Autodesk Inventor part; units mm, degrees
ref_plane "YZ Plane" through (0, 0, 0) normal (1, 0, 0) x (0, 1, 0)
ref_plane "XZ Plane" through (0, 0, 0) normal (0, 1, 0) x (-1, 0, 0)
ref_plane "XY Plane" through (0, 0, 0) normal (0, 0, 1) x (1, 0, 0)
sketch "Sketch1" plane through (0, 0, 0) normal (0, 1, 0) x (-1, 0, 0)
  line L0 (0, -23.3131) -> (0, 24.6505)
  line L1 (49.2542, 0) -> (-47.6933, 0)
  arc A0 (37.265, -6.345) -> (37.265, -10.765) centre (35.3109, -8.555) ccw
  line L2 (37.265, -14.815) -> (37.265, -10.765)
  arc A1 (37.265, 10.765) -> (37.265, 6.345) centre (35.3109, 8.555) ccw
  line L3 (37.265, 14.815) -> (37.265, 10.765)
  line L4 (37.265, -6.345) -> (37.265, 6.345)
  line L5 (37.265, -14.815) -> (29.695, -14.815)
  line L6 (37.265, 14.815) -> (29.695, 14.815)
  arc A2 (-37.265, -10.765) -> (-37.265, -6.345) centre (-35.3109, -8.555) ccw
  line L7 (-37.265, -14.815) -> (-37.265, -10.765)
  line L8 (-37.265, 14.815) -> (-37.265, 10.765)
  arc A3 (-37.265, 6.345) -> (-37.265, 10.765) centre (-35.3109, 8.555) ccw
  line L9 (-37.265, -6.345) -> (-37.265, 6.345)
  line L10 (-37.265, -14.815) -> (-29.695, -14.815)
  line L11 (-37.265, 14.815) -> (-29.695, 14.815)
  line L12 (29.695, -14.815) -> (-29.695, -14.815)
  line L13 (-29.695, 14.815) -> (29.695, 14.815)
  line L14 (29.695, -14.815) -> (29.695, 14.815)
  line L15 (-29.695, -14.815) -> (-29.695, 14.815)
  point P0 (0, 0)
  dimension "d3" = 4.42
  dimension "d6" = 2.95
  dimension "d7" = 7.57
  dimension "d8" = 3.31
  dimension "d9" = 59.39
  dimension "d10" = 29.63
extrude "Extrusion1" add sketch "Sketch1" along normal blind 3.95
sketch "Sketch2" plane through (0, 3.95, 0) normal (0, 1, 0) x (1, 0, 0)
  line L0 (37.265, 14.815) -> (-37.265, 14.815)
  line L1 (-37.265, -14.815) -> (37.265, -14.815)
  line L2 (-29.695, 14.815) -> (29.695, 14.815)
  line L3 (29.695, 14.815) -> (29.695, -14.815)
  line L4 (29.695, -14.815) -> (-29.695, -14.815)
  line L5 (-29.695, -14.815) -> (-29.695, 14.815)
  point P0 (0, 0)
  dimension "d13" = 59.39
  dimension "d14" = 29.695
extrude "Extrusion2" add sketch "Sketch2" along normal blind 3.5
sketch "Sketch3" plane through (0, 0, 0) normal (0, -1, 0) x (1, 0, 0)
  line L0 (37.265, -14.815) -> (-37.265, -14.815)
  line L1 (-37.265, 14.815) -> (37.265, 14.815)
  line L2 (-29.695, 14.815) -> (29.695, 14.815)
  line L3 (29.695, 14.815) -> (29.695, -14.815)
  line L4 (29.695, -14.815) -> (-29.695, -14.815)
  line L5 (-29.695, -14.815) -> (-29.695, 14.815)
  point P0 (0, 0)
  dimension "d17" = 59.39
  dimension "d18" = 29.695
extrude "Extrusion3" add sketch "Sketch3" along normal blind 49.69
sketch "Sketch4" plane through (37.265, 0, 14.815) normal (0, 0, 1) x (1, 0, 0)
  line L0 (-7.57, -49.69) -> (-66.96, -49.69)
  line L1 (-66.96, 7.45) -> (-7.57, 7.45)
  line L2 (-74.53, 0) -> (-74.53, 3.95)
  line L3 (-66.96, 7.45) -> (-55.11, 10.31)
  line L4 (-55.11, 10.31) -> (-19.42, 10.31)
  line L5 (-19.42, 10.31) -> (-7.57, 7.45)
  line L6 (14.6439, 12.17) -> (-93.8376, 12.17) construction
  line L7 (-75.1527, 11.11) -> (-5.1295, 11.11) construction
  point P0 (-37.265, 0)
  dimension "d21" = 11.85
  dimension "d22" = 11.85
  dimension "d31" = 1.06
  dimension "d32" = 0.8
  dimension "d44" = 60.8
sketch "Sketch5" plane through (0, 7.45, 0) normal (0, 1, 0) x (1, 0, 0)
  line L0 (29.695, -14.815) -> (29.695, 14.815)
  line L1 (29.695, 14.815) -> (-29.695, 14.815)
  circle A0 centre (17.845, 0) radius 9
  point P0 (0, 0)
  dimension "d23" = 11.85
  dimension "d24" = 18
  dimension "d29" = 14.815
extrude "Extrusion4" add sketch "Sketch5" along normal blind 4.72
sketch "Sketch6" plane through (0, 7.45, 0) normal (0, 1, 0) x (1, 0, 0)
  line L0 (-29.695, 14.815) -> (-29.695, -14.815)
  line L1 (-22.695, 12.5) -> (3.505, 12.5)
  line L2 (3.505, 12.5) -> (3.505, -12.5)
  line L3 (3.505, -12.5) -> (-22.695, -12.5)
  line L4 (-22.695, -12.5) -> (-22.695, 12.5)
  line L5 (-37.265, 6.345) -> (-37.265, -6.345)
  point P0 (0, 0)
  dimension "d35" = 25
  dimension "d36" = 12.5
  dimension "d38" = 26.2
  dimension "d39" = 7
extrude "Extrusion5" add sketch "Sketch6" along normal blind 3.66
extrude "Extrusion6" add sketch "Sketch4" against normal up to surface (29.63 mm away)
sketch "Sketch7" plane through (17.845, 12.17, 0) normal (0, 1, 0) x (1, 0, 0)
  circle A0 centre (0, 0) radius 9
  circle A1 centre (0, 0) radius 3.365
  point P0 (-17.845, 0)
  dimension "d45" = 6.73
extrude "Extrusion7" add sketch "Sketch7" along normal blind 5.95 contours A1
chamfer "Chamfer1" distance 0.25 distance2 2.2 1 edges at (0, -49.69, -14.815) measured on face at (-9.8983, -49.69, 4.9383)
chamfer "Chamfer2" distance 0.25 distance2 2.2 1 edges at (0, -49.69, 14.815) measured on face at (9.8983, -49.69, -4.7717)
chamfer "Chamfer3" distance 0.25 distance2 2.2 1 edges at (29.695, -49.69, 0) measured on face at (-9.8983, -49.69, 4.855)
chamfer "Chamfer4" distance 0.25 distance2 2.2 1 edges at (-29.695, -49.69, 0) measured on face at (-9.9817, -49.69, 4.855)
equation "\"d13\" = d9"
equation "\"d17\" = d9"
equation "\"d22\" = d21"
equation "\"d29\" = 0.5 * d10"
properties part number "ServoModel"
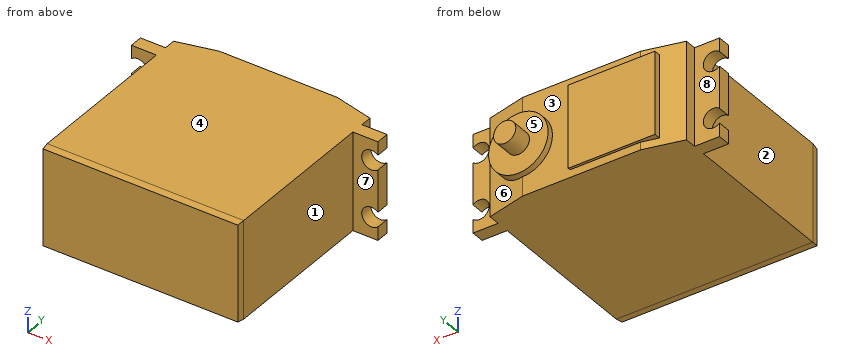
Geometry check sheet. Reference: the model listing, model coordinates, mm. Face numbers are marked on the shaded views. A direction names the side the tool comes from. Round coordinates to 2 decimals unless told otherwise and drop trailing zeros. Loops run counter-clockwise (first coordinate to the right, second up) from the corner with the lowest first, then second, coordinate; pieces in that order, holes last. Notation, with made-up numbers: (-4.5, -19.75) - (21.5, -19.75) arc R8 cw to (21.5, -11.75) - close; hole circle Ø4 at (83, 41.25). An arc over 180 degrees is marked (long way). Write each question's results on one line, items separated by ' | '. Start each with the question number.
Q1. Cross-section at A-A on z = 0. Enter the section's corners in (x, y) (3 decimals), and give its area (3 significant figures).
Q2. Cross-section at D-D on z = 7.5. Enter the section's corners in (x, y) (3 decimals).
Q3. Gauge pin test, flat ends, axial feed: P1, Ø12, axis at x = 7, z = 1.5, coming from the +Y side; P2, Ø6, axis at x = 34.5, z = -0.5, coming from the +Y side; P3, Ø9, axis at y = -25, z = -1.5, coming from the -X side (3 decimals). Record the tip position at first contact, or that the pin passes through.
Q4. Release check for a two-part mould opening along X. For the marked faces 1, 2, 3 and 4 record: +X half, -X half, draft (parallel to the pull), parting line (faces both ways), or undercut.
Q5. Cross-section at C-C on y = 1. Enter the section's corners in (x, z) (3 decimals).
Q6. Access from +Z, -Z, +X, -X, +Y, -Y to the whole of each face (thin tool, end or side, straight path). Record for the marked faces 5, 6, 7 and 8.
Q7. Thickness scan on line 1 (Y direction, x = 4, z = -12); line 2 (X direction, y = -27.5, z = -5) (3 decimals); line 3 (Y direction, x = 20, z = -6.75). Record the ranges inside material, lowest first. Write a range as [from, to].
Q8. Cross-section at B-B on x = -10. Enter the section's corners in (y, z) (3 decimals), and give its area (3 significant figures).
Answers below:
1) outline: (-37.265, 0) - (-29.695, 0) - (-29.695, -47.49) - (-29.445, -49.69) - (29.445, -49.69) - (29.695, -47.49) - (29.695, 0) - (37.265, 0) - (37.265, 3.95) - (29.695, 3.95) - (29.695, 7.45) - (26.845, 8.138) - (26.845, 12.17) - (21.21, 12.17) - (21.21, 18.12) - (14.48, 18.12) - (14.48, 12.17) - (8.845, 12.17) - (8.845, 10.31) - (3.505, 10.31) - (3.505, 11.11) - (-22.695, 11.11) - (-22.695, 9.139) - (-29.695, 7.45) - (-29.695, 3.95) - (-37.265, 3.95) - close | area: 3,700 mm²
2) outline: (-32.556, 0) - (-29.695, 0) - (-29.695, -47.49) - (-29.445, -49.69) - (29.445, -49.69) - (29.695, -47.49) - (29.695, 0) - (32.556, 0) - (32.556, 3.95) - (29.695, 3.95) - (29.695, 7.45) - (22.82, 9.109) - (22.82, 12.17) - (12.87, 12.17) - (12.87, 10.31) - (3.505, 10.31) - (3.505, 11.11) - (-22.695, 11.11) - (-22.695, 9.139) - (-29.695, 7.45) - (-29.695, 3.95) - (-32.556, 3.95) - close
3) P1: stops at y = 12.17 | P2: stops at y = 3.95 | P3: stops at x = -29.695
4) face 1: +X half | face 2: -X half | face 3: undercut | face 4: draft
5) outline: (-37.265, -14.815) - (37.265, -14.815) - (37.265, -10.765) arc R2.95 cw (long way) to (37.265, -6.345) - (37.265, 6.345) arc R2.95 cw (long way) to (37.265, 10.765) - (37.265, 14.815) - (-37.265, 14.815) - (-37.265, 10.765) arc R2.95 cw (long way) to (-37.265, 6.345) - (-37.265, -6.345) arc R2.95 cw (long way) to (-37.265, -10.765) - close
6) face 5: +Y | face 6: +X, +Y | face 7: +Z, -Z, +X, -Y | face 8: +Z, -Z, -X, +Y
7) line 1: y = [-49.69, 10.31] | line 2: x = [-29.695, 29.695] | line 3: y = [-49.69, 12.17]
8) outline: (-49.69, -14.565) - (-47.49, -14.815) - (10.31, -14.815) - (10.31, -12.5) - (11.11, -12.5) - (11.11, 12.5) - (10.31, 12.5) - (10.31, 14.815) - (-47.49, 14.815) - (-49.69, 14.565) - close | area: 1,800 mm²
